For this review, use the dimensioned drawing (mm, ordinates from the lowest corner) and the shaded views. Coordinates: 2 decimals unless noted, no trailing zeros. Write each loop counter-clockwise with the first axis right and the second up, starting at its lowest first coordinate (ties: lowest second). Pieces come first, ordered by that corner, then holes. Notation, with made-up numbers: M 74.5,-17 L 103.5,-17 A20 ccw 103.5,6 Z; hole C 34,29.25 d8. An arc over 180 degrees is marked long. One line per question, with ' | ' between items.
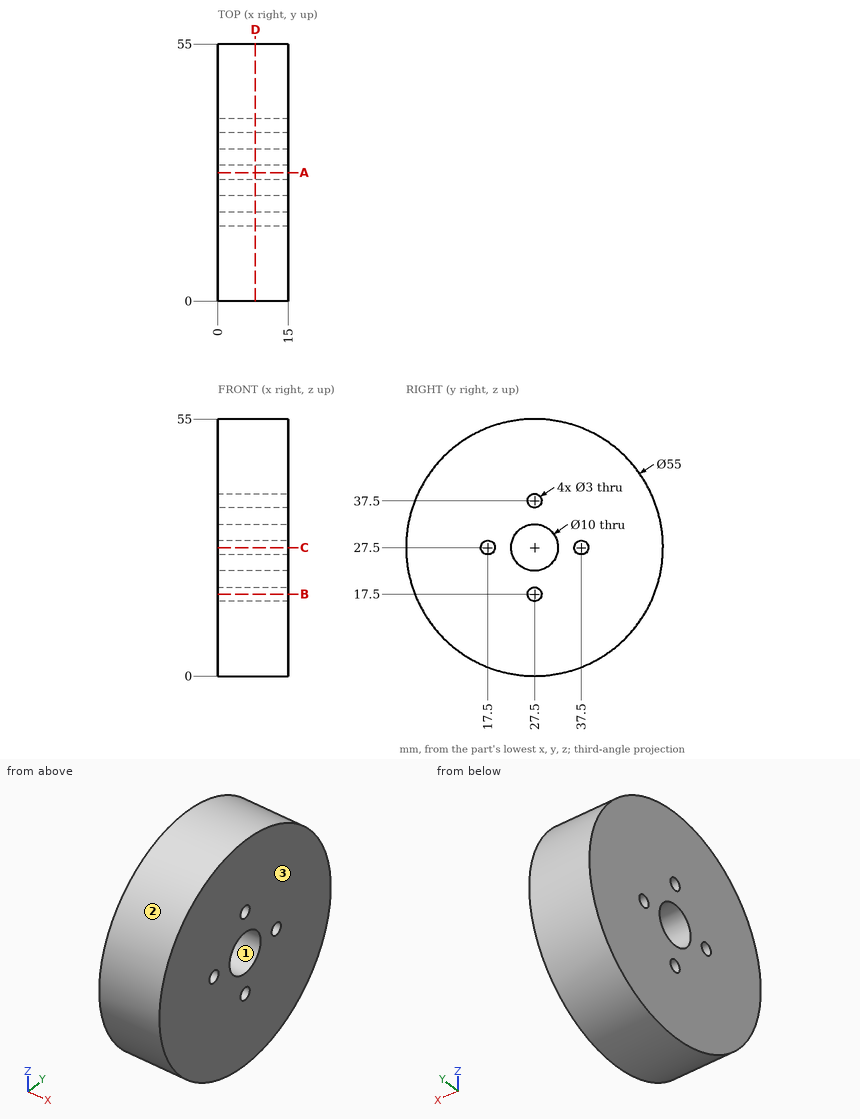
1. Draft analysis for pull direction Y (two halves, no side actions). For the marked faces 1, 2 and 3, state which applies: pulls with the +Y half, pulls with the -Y half, needs draft (parallel to the pull), parting line crosses it, or undercut.
Answer sheet:
face 1: undercut | face 2: parting line crosses it | face 3: needs draft
2. Take a section at D-D (x = 8). Write out the cut boundary in (y, z).
Answer sheet:
outline: C 27.5,27.5 d55; hole C 17.5,27.5 d3; hole C 27.5,27.5 d10; hole C 27.5,17.5 d3; hole C 27.5,37.5 d3; hole C 37.5,27.5 d3
3. Insertion check: pin 1 Ø5 at (x, z) = (4, 32.5) entering from +Y; pin 2 Ø1.8 at (y, z) = (27.5, 37.5) entering from +X; pin 3 Ø5 at (x, z) = (8.5, 33.5) entering from +Y; pin 4 Ø3 at (x, y) = (10.5, 31.5) entering from +Z. Each pin has a flat end and moves straight along its axis. Give the tip position at first contact, or say it passes through.
Answer sheet:
pin 1: y = 54.89 | pin 2: through | pin 3: y = 54.78 | pin 4: z = 54.89
4. To check wall thickness, follow line 1 along Y through (x, z) = (10.75, 27.5); line 2 along Z through (x, y) = (2.5, 30.5); line 3 along Y through (x, z) = (8.5, 37.5). State the ranges of each line that lie inside material, in increasing order. Write a range as [from, to].
Answer sheet:
line 1: [0, 16], [19, 22.5], [32.5, 36], [39, 55] | line 2: [0.16, 23.5], [31.5, 54.84] | line 3: [1.88, 26], [29, 53.12]
5. Take a section at B-B (z = 17.5). Write out the cut boundary in (x, y), then the cut area to 3 significant figures.
Answer sheet:
outline: M 0,1.88 L 15,1.88 L 15,26 L 0,26 Z; M 0,29 L 15,29 L 15,53.12 L 0,53.12 Z | area: 724 mm^2
6. Take a section at A-A (y = 27.5). Write out the cut boundary in (x, z).
Answer sheet:
outline: M 0,0 L 15,0 L 15,16 L 0,16 Z; M 0,19 L 15,19 L 15,22.5 L 0,22.5 Z; M 0,32.5 L 15,32.5 L 15,36 L 0,36 Z; M 0,39 L 15,39 L 15,55 L 0,55 Z
